from build123d import *

# Parameters (mm, degrees)
F0_W      = 110
F0_H      = 130
F1_DEPTH  = 20
F2_W      = 100
F2_H      = 120
F3_DEPTH  = 17
F4_W      = 100
F4_H      = 2.5
F5_DEPTH  = 17
F6_SIZE   = 5
F7_SIZE   = 2
F8_R      = 7
F9_R      = 5
F10_R     = 5
F11_R     = 5
F12_W     = 5
F12_H     = 77.5
F13_DEPTH = 5.1
F14_W     = 5
F14_H     = 13
F15_DEPTH = 5.1


with BuildPart() as f1:
    # F0 (on Front) → F1 (new body)
    with BuildSketch(Plane.XZ):
        Rectangle(F0_W, F0_H)
    extrude(amount=F1_DEPTH)

    # F2 (on face) → F3 (cut)
    with BuildSketch(Plane.XZ.offset(20)):
        Rectangle(F2_W, F2_H)
    extrude(amount=-F3_DEPTH, mode=Mode.SUBTRACT)

    # F4 (on face) → F5 (join, through all)
    with BuildSketch(Plane.XZ.offset(3)):
        with Locations((0, 38.75)):
            Rectangle(F4_W, F4_H)
    extrude(amount=F5_DEPTH)

    # F6
    f6_edges = [f1.edges().sort_by_distance(p)[0] for p in [
        (55, -10, 65),
        (-55, -10, 65),
        (55, -10, -65),
        (-55, -10, -65),
    ]]
    chamfer(f6_edges, length=F6_SIZE)

    # F7
    f7_edges = [f1.edges().sort_by_distance(p)[0] for p in [
        (50, -11.5, 60),
        (-50, -11.5, 60),
    ]]
    chamfer(f7_edges, length=F7_SIZE)

    # F8
    f8_edges = [f1.edges().sort_by_distance(p)[0] for p in [
        (0, 0, -65),
        (-52.5, 0, -62.5),
        (52.5, 0, -62.5),
        (-55, 0, 0),
        (55, 0, 0),
        (-52.5, 0, 62.5),
        (52.5, 0, 62.5),
        (0, 0, 65),
    ]]
    fillet(f8_edges, radius=F8_R)

    # F9
    f9_edges = [f1.edges().sort_by_distance(p)[0] for p in [
        (-55, -13.5, -60),
        (-50, -13.5, -65),
        (55, -13.5, -60),
        (50, -13.5, -65),
        (50, -13.5, 65),
        (55, -13.5, 60),
    ]]
    fillet(f9_edges, radius=F9_R)

    # F10
    f10_edges = [f1.edges().sort_by_distance(p)[0] for p in [
        (-50, -13.5, 65),
        (-55, -13.5, 60),
    ]]
    fillet(f10_edges, radius=F10_R)

    # F11
    f11_edges = [f1.edges().sort_by_distance(p)[0] for p in [
        (-50, -11.5, -60),
        (50, -11.5, -60),
    ]]
    fillet(f11_edges, radius=F11_R)

    # F12 (on face) → F13 (cut)
    with BuildSketch(Plane.XZ.offset(20)):
        with Locations((52.5, -11.25)):
            Rectangle(F12_W, F12_H)
    extrude(amount=-F13_DEPTH, mode=Mode.SUBTRACT)

    # F14 (on face) → F15 (cut)
    with BuildSketch(Plane.XZ.offset(20)):
        with Locations((52.5, 49.5)):
            Rectangle(F14_W, F14_H)
    extrude(amount=-F15_DEPTH, mode=Mode.SUBTRACT)


solid = f1.part
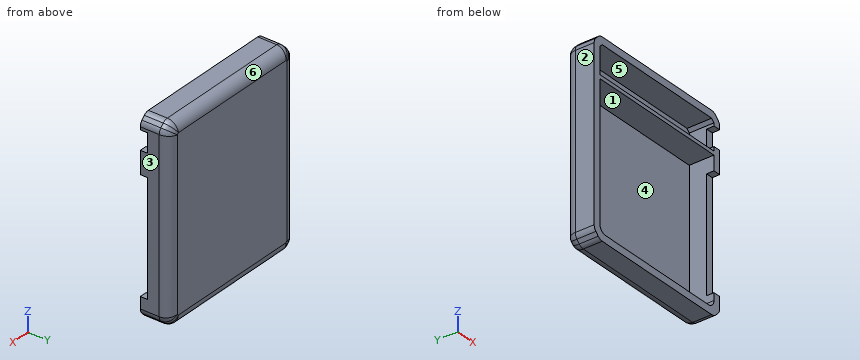
The listing builds one solid part. Answer for the finished solid, in the listing's coordinates (mm). Face numbers are marked on the shaded views. A direction names the side the tool comes from. Give positions to 0.01 mm unless a question says otherwise; leave off trailing zeros. Order: outer loops, then holes, each group sorted by start corner. A loop starts at its lowest first (then second) coordinate and runs counter-clockwise, first axis right, second up. Notation, with made-up numbers: (-40, 63) - (-26, 63) arc R21 ccw to (-26, 87) - close; hole circle Ø6 at (60, -7.75). An arc over 180 degrees is marked (long way). Use one line per item in the form item = value.
1) Find section A-A on x = -24. Determine the outline of the cut face in (y, z), and give its area (3 significant figures).
Verdict:
outline = (-20, -65) - (-7, -65) arc R7 ccw to (0, -58) - (0, 58) arc R7 ccw to (-7, 65) - (-20, 65) - (-20, 60) - (-3, 60) - (-3, 40) - (-20, 40) - (-20, 37.5) - (-3, 37.5) - (-3, -60) - (-20, -60) - close
area = 581 mm^2
2) The mould has two halves that part along X. Classify the marked faces 3, 4, 5 and 6: released by +X, released by -X, zero draft, split by the parting line, or undercut.
Verdict:
face_3 = released by +X
face_4 = undercut
face_5 = undercut
face_6 = zero draft
3) Consider probe 1 along Z at (x, y) = (-36, -9.75); probe 2 along X at (y, z) = (-10.25, 58); probe 3 along Z at (x, y) = (-3.5, -3.75). Determine where each line is inside the solid, lowest interval first. Write a range as [from, to].
Verdict:
probe_1 = [-65, -60], [37.5, 40], [60, 65]
probe_2 = [-55, -50], [50, 55]
probe_3 = [-64.2, -60], [37.5, 40], [60, 64.2]
4) Each of these flat-tipped pins is pushed along its axis until it touches: pin 1 (4 mm diameter, centred on x = 53, y = -18.5, fed in from +Z); pin 2 (1.5 mm diameter, centred on y = -16, z = -10, fed in from +X); pin 3 (5.5 mm diameter, centred on x = 53.5, y = -18.5, fed in from -Z). Where does it stop, or does it pass through?
Verdict:
pin_1 = 63.95
pin_2 = -50
pin_3 = -64.13
5) Find section B-B on y = -10.25. Determine the outline of the cut face in (x, z), and give its area (3 significant figures).
Verdict:
outline = (-55, -57.93) arc R5 ccw to (-53.54, -61.46) - (-51.46, -63.54) arc R5 ccw to (-47.93, -65) - (47.93, -65) arc R5 ccw to (51.46, -63.54) - (53.54, -61.46) arc R5 ccw to (55, -57.93) - (55, 57.93) arc R5 ccw to (53.54, 61.46) - (51.46, 63.54) arc R5 ccw to (47.93, 65) - (-47.93, 65) arc R5 ccw to (-51.46, 63.54) - (-53.54, 61.46) arc R5 ccw to (-55, 57.93) - close; hole (-50, -55) arc R5 ccw to (-45, -60) - (45, -60) arc R5 ccw to (50, -55) - (50, 37.5) - (-50, 37.5) - close; hole (-50, 40) - (50, 40) - (50, 58) - (48, 60) - (-48, 60) - (-50, 58) - close
area = 2,510 mm^2
6) Find section C-C on z = -27.5. Determine the outline of the cut face in (x, y).
Verdict:
outline = (-55, -20) - (-50, -20) - (-50, -3) - (50, -3) - (50, -14.9) - (55, -14.9) - (55, -7) arc R7 ccw to (48, 0) - (-48, 0) arc R7 ccw to (-55, -7) - close
7) For the marked faces 1 and 2, determine the directions among +Z, -Z, +X, -X, +Y, -Y from which every point of the face is accessible in a straight line to the end or side of a thin tool.
Verdict:
face_1 = -Y
face_2 = +Z, -Z, -X, +Y, -Y
